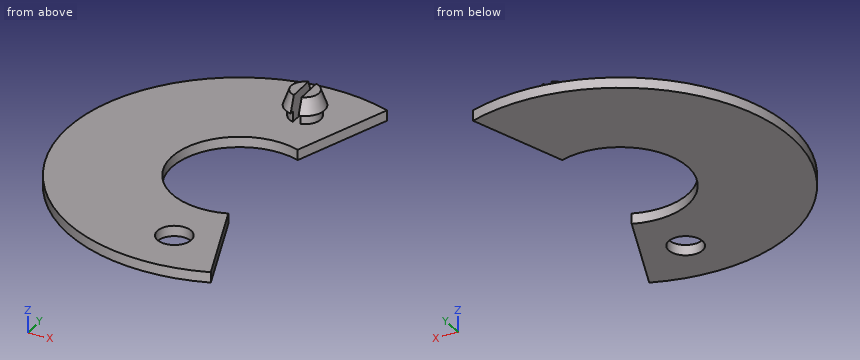
```python
from build123d import *

# Parameters (mm, degrees)
F0_R     = 3.25
F0_R_2   = 3
F1_DEPTH = 2
F2_DEPTH = 4
F3_R     = 3.75
F3_R_2   = 3
F4_DEPTH = 3
F4_TAPER = 20
F6_DEPTH = 5


with BuildPart() as f1:
    # F0 (on Top) → F1 (new body)
    with BuildSketch(Plane.XY):
        with BuildLine():
            ThreePointArc((4.4462618632, -12.2160040702), (-13, 0), (4.4462618632, 12.2160040702))
            Line((4.4462618632, 12.2160040702), (11.2866647297, 31.0098564859))
            ThreePointArc((11.2866647297, 31.0098564859), (-33, 0), (11.2866647297, -31.0098564859))
            Line((11.2866647297, -31.0098564859), (4.4462618632, -12.2160040702))
        make_face()
        with Locations((0, -23)):
            Circle(F0_R, mode=Mode.SUBTRACT)
        with Locations((0, 23)):
            Circle(F0_R_2, mode=Mode.SUBTRACT)
    extrude(amount=F1_DEPTH)

    # F0 (on Top) → F2 (join)
    with BuildSketch(Plane.XY):
        with Locations((0, 23)):
            Circle(F0_R_2)
    extrude(amount=F2_DEPTH)

    # F3 (on face) → F4 (join)
    with BuildSketch(Plane.XY.offset(4)):
        with Locations((0, 23)):
            Circle(F3_R)
        with Locations((0, 23)):
            Circle(F3_R_2, mode=Mode.SUBTRACT)
        with Locations((0, 23)):
            Circle(F3_R_2)
    extrude(amount=F4_DEPTH, taper=F4_TAPER)

    # F5 (on face) → F6 (cut)
    with BuildSketch(Plane.XY.offset(7)):
        with BuildLine():
            ThreePointArc((0.75, 20.4499139795), (0, 20.3419107028), (-0.75, 20.4499139795))
            Line((-0.75, 20.4499139795), (-0.75, 18.6920836568))
            Line((-0.75, 18.6920836568), (0.75, 18.7304485589))
            Line((0.75, 18.7304485589), (0.75, 20.4499139795))
        make_face()
        with BuildLine():
            ThreePointArc((0.75, 25.5500860205), (0, 25.6580892972), (-0.75, 25.5500860205))
            Line((-0.75, 25.5500860205), (-0.75, 20.4499139795))
            ThreePointArc((-0.75, 20.4499139795), (0, 20.3419107028), (0.75, 20.4499139795))
            Line((0.75, 20.4499139795), (0.75, 25.5500860205))
        make_face()
        with BuildLine():
            Line((-0.75, 27.6506636292), (-0.75, 25.5500860205))
            ThreePointArc((-0.75, 25.5500860205), (0, 25.6580892972), (0.75, 25.5500860205))
            Line((0.75, 25.5500860205), (0.75, 27.6890285313))
            Line((0.75, 27.6890285313), (-0.75, 27.6506636292))
        make_face()
    extrude(amount=-F6_DEPTH, mode=Mode.SUBTRACT)


solid = f1.part
```
Geometry: final body of the model. Coordinates: model frame, mm. Round coordinates to 2 decimals unless told otherwise and drop trailing zeros. Order: outer loops, then holes, each group sorted by start corner. A loop starts at its lowest first (then second) coordinate and runs counter-clockwise, first axis right, second up. Notation, with made-up numbers: (-9.75, -36) -> (22.25, -36) arc R17 cw to (22.25, -20) -> close; hole circle Ø5 at (89.25, 11.25). An arc over 180 degrees is marked (long way). Use one line per item in the form item = value. Start each with the question number.
1. Cut plane D-D (y = 0). Return the cut outline in (x, z).
2. Pin query (flat end, axial travel): pin 1 Ø22 at (x, y) = (-6.5, 2.5) entering from +Z; pin 2 Ø4 at (y, z) = (24, 5) entering from -X; pin 3 Ø3 at (y, z) = (-15, 3) entering from -X. Return the tip coordinate at first contact, or that it passes through.
3. Cut plane B-B (y = -23). Return the cut outline in (x, z).
4. Cut plane A-A (x = 0). Return the cut outline in (y, z), then the cut area to 3 significant figures.
5. Cut plane C-C (z = 3). Return the cut outline in (x, y), then the cut area to 3 significant figures.
6. Line query: probe 1 along Y at (x, z) = (0, 1.1); probe 2 along Y at (x, z) = (-4, 1.25); probe 3 along Z at (x, y) = (-21.5, -1.5). Output: solid intervals per line, ascending.
Solution:
q1.outline = (-33, 0) -> (-13, 0) -> (-13, 2) -> (-33, 2) -> close
q2.pin_1 = 2
q2.pin_2 = -3.75
q2.pin_3 = -29.94
q3.outline = (-23.66, 0) -> (-3.25, 0) -> (-3.25, 2) -> (-23.66, 2) -> close; (3.25, 0) -> (8.37, 0) -> (8.37, 2) -> (3.25, 2) -> close
q4.outline = (-33, 0) -> (-26.25, 0) -> (-26.25, 2) -> (-33, 2) -> close; (-19.75, 0) -> (-13, 0) -> (-13, 2) -> (-19.75, 2) -> close; (13, 0) -> (33, 0) -> (33, 2) -> (13, 2) -> close
q4.area = 67.0 mm^2
q5.outline = (-0.75, 20.1) -> (-0.75, 25.9) arc R3 ccw to start; (0.75, 20.1) arc R3 ccw to (0.75, 25.9) -> close
q5.area = 19.4 mm^2
q6.probe_1 = -33 to -26.25, -19.75 to -13, 13 to 33
q6.probe_2 = -32.76 to -12.37, 12.37 to 32.76
q6.probe_3 = 0 to 2
